Verification items for the finished model (mm, model axes). A direction names the side the tool comes from. Coordinates: 2 decimals unless noted, no trailing zeros. Loops run counter-clockwise (first coordinate to the right, second up) from the corner with the lowest first, then second, coordinate; pieces in that order, holes last. Notation, with made-up numbers: (-10, 80.25) - (4, 80.25) arc R37 cw to (4, 116.25) - close; hole circle Ø8 at (-24, -6). An arc over 180 degrees is marked (long way). One line per item, written item: value. Start each with the question number.
(1) Section check B-B (z = 5.5). Record the boundary of the cut face in (x, y), plus the area to 3 significant figures.
(2) Section check D-D (z = 1). Record the boundary of the cut face in (x, y).
(3) Gauge pin test, flat ends, axial feed: P1, Ø10, axis at x = 10.5, z = -14, coming from the +Y side; P2, Ø3, axis at x = -11.5, y = 1, coming from the -Z side; P3, Ø1.2, axis at y = 0, z = 12, coming from the -X side; P4, Ø1.5, axis at x = -20.06, y = 6.5, coming from the +Z side (3 decimals). Record the tip position at first contact, or that the pin passes through.
(4) Section check A-A (y = 6.5). Record the boundary of the cut face in (x, z), plus the area to 3 significant figures.
(5) Thickness scan on probe 1 along Z at (x, y) = (-10, 7); probe 2 along Y at (x, z) = (-4.5, -14.5); probe 3 along Y at (x, z) = (-20.06, 16.75). Record the ranges inside material, lowest first. Write a range as [from, to].
(6) Section check C-C (x = -6.8). Record the boundary of the cut face in (y, z), plus the area to 3 significant figures.
(7) Draft check along Z on faces 1 (the face through (-11, 0, -2.9)), 2 (the face through (-6.8, 9, -16.4)), 3 (the face through (-11, 0, 9.1)). Enter one of: +Z half, -Z half, draft (parallel to the pull), parting line (faces both ways), or undercut.
(8) Set-up check for faces 4 (the face through (-11, 0, 2.9)), 5 (the face through (-9, 4.7, -1)), 6 (the face through (-4, 7.9, 16)), 7 (the face through (-13, 7.9, 16)): record each of +Z, -Z, +X, -X, +Y, -Y from which the full face is reachable in a straight line by a thin tool's end or side.
```python
from build123d import *
from build123d.topology import SkipClean

# Parameters (mm, degrees)
EXTRUDE_1_DEPTH     = 18.5
SKETCH_2_W          = 6
SKETCH_2_H          = 5.8
SKETCH_2_H_2        = 9.4
SKETCH_2_W_2        = 12
SKETCH_2_H_3        = 20.2
CUT_EXTRUDE_1_DEPTH = 25.150569351
EXTRUDE_2_REACH     = 41.975
SKETCH_4_R          = 0.85
SKETCH_5_W          = 27.2
SKETCH_5_H          = 4.3
CUT_EXTRUDE_2_DEPTH = 43.825268242
SKETCH_6_W          = 27.2
SKETCH_6_H          = 0.5
CUT_EXTRUDE_3_DEPTH = 2


with BuildPart() as part:
    # 草图1 → 凸台-拉伸1 (new, symmetric)
    with BuildSketch(Plane.XY):
        with BuildLine():
            ThreePointArc((-11, 0), (-11.585786438, 1.414213562), (-13, 2))
            Line((-13, 2), (-13, 1.15))
            ThreePointArc((-13, 1.15), (-12.186827202, 0.813172798), (-11.85, 0))
            ThreePointArc((-11.85, 0), (-12.186827202, -0.813172798), (-13, -1.15))
            Line((-13, -1.15), (-13, -2))
            ThreePointArc((-13, -2), (-11.585786438, -1.414213562), (-11, 0))
        make_face()
        with BuildLine():
            Line((-13, 1.15), (-13, 2))
            ThreePointArc((-13, 2), (-15, 0), (-13, -2))
            Line((-13, -2), (-13, -1.15))
            ThreePointArc((-13, -1.15), (-14.15, 0), (-13, 1.15))
        make_face()
        with BuildLine():
            ThreePointArc((-11, 0), (-11.585786438, 1.414213562), (-13, 2))
            Line((-13, 2), (-13, 1.15))
            ThreePointArc((-13, 1.15), (-12.186827202, 0.813172798), (-11.85, 0))
            ThreePointArc((-11.85, 0), (-12.186827202, -0.813172798), (-13, -1.15))
            Line((-13, -1.15), (-13, -2))
            ThreePointArc((-13, -2), (-11.585786438, -1.414213562), (-11, 0))
        make_face()
        with BuildLine():
            Line((-13, 1.15), (-13, 2))
            ThreePointArc((-13, 2), (-15, 0), (-13, -2))
            Line((-13, -2), (-13, -1.15))
            ThreePointArc((-13, -1.15), (-14.15, 0), (-13, 1.15))
        make_face()
        with BuildLine():
            Line((13, 2), (-13, 2))
            ThreePointArc((-13, 2), (-11.585786438, 1.414213562), (-11, 0))
            ThreePointArc((-11, 0), (-11.585786438, -1.414213562), (-13, -2))
            Line((-13, -2), (13, -2))
            ThreePointArc((13, -2), (11, 0), (13, 2))
        make_face()
        with BuildLine():
            ThreePointArc((15, 0), (14.414213562, 1.414213562), (13, 2))
            Line((13, 2), (13, 1.15))
            ThreePointArc((13, 1.15), (13.813172798, 0.813172798), (14.15, 0))
            ThreePointArc((14.15, 0), (13.813172798, -0.813172798), (13, -1.15))
            Line((13, -1.15), (13, -2))
            ThreePointArc((13, -2), (14.414213562, -1.414213562), (15, 0))
        make_face()
        with BuildLine():
            Line((13, 1.15), (13, 2))
            ThreePointArc((13, 2), (11, 0), (13, -2))
            Line((13, -2), (13, -1.15))
            ThreePointArc((13, -1.15), (11.85, 0), (13, 1.15))
        make_face()
        with BuildLine():
            ThreePointArc((15, 0), (14.414213562, 1.414213562), (13, 2))
            Line((13, 2), (13, 1.15))
            ThreePointArc((13, 1.15), (13.813172798, 0.813172798), (14.15, 0))
            ThreePointArc((14.15, 0), (13.813172798, -0.813172798), (13, -1.15))
            Line((13, -1.15), (13, -2))
            ThreePointArc((13, -2), (14.414213562, -1.414213562), (15, 0))
        make_face()
        with BuildLine():
            Line((13, 1.15), (13, 2))
            ThreePointArc((13, 2), (11, 0), (13, -2))
            Line((13, -2), (13, -1.15))
            ThreePointArc((13, -1.15), (11.85, 0), (13, 1.15))
        make_face()
    extrude(amount=EXTRUDE_1_DEPTH, both=True)

    # 草图2 → 切除-拉伸1 (cut, through all)
    with SkipClean():  # the faces are left unmerged after this step: merging them gives an invalid solid
        with BuildSketch(Plane(origin=(0, 2, 0), x_dir=(1, 0, 0), z_dir=(0, 1, 0))):
            with Locations((-12, 0)):
                Rectangle(SKETCH_2_W, SKETCH_2_H)
            with Locations((-12, -13.8)):
                Rectangle(SKETCH_2_W, SKETCH_2_H_2)
            with Locations((-12, 13.8)):
                Rectangle(SKETCH_2_W, SKETCH_2_H_2)
            with Locations((9, 0)):
                Rectangle(SKETCH_2_W_2, SKETCH_2_H_3)
        extrude(amount=-CUT_EXTRUDE_1_DEPTH, mode=Mode.SUBTRACT)

    # 凸台-拉伸2: up to this face of the body (flat: up to its plane)
    extrude_2_end = Plane(part.part.faces().sort_by_distance((2.318945453, 0, -18.5))[0])
    # 草图4 → 凸台-拉伸2 (add, up to the picked face)
    with BuildSketch(Plane.XY.offset(18.5), mode=Mode.PRIVATE) as extrude_2_sk1:
        with BuildLine():
            Line((-10.789828689, 2.382780472), (-9, 2))
            Line((-9, 2), (8, 2))
            Line((8, 2), (-3.8, 7.9))
            Line((-3.8, 7.9), (-4.728768482, 7.9))
            ThreePointArc((-4.728768482, 7.9), (-6.8, 9), (-8.871231518, 7.9))
            Line((-8.871231518, 7.9), (-17.988768482, 7.9))
            ThreePointArc((-17.988768482, 7.9), (-20.06, 9), (-22.131231518, 7.9))
            Line((-22.131231518, 7.9), (-22.56, 7.9))
            Line((-22.56, 7.9), (-22.56, 4.9))
            Line((-22.56, 4.9), (-14.042229791, 3.078352979))
            ThreePointArc((-14.042229791, 3.078352979), (-12.320311008, 3.178131979), (-10.789828689, 2.382780472))
        make_face()
        with Locations((-20.06, 6.5)):
            Circle(SKETCH_4_R, mode=Mode.SUBTRACT)
        with Locations((-6.8, 6.5)):
            Circle(SKETCH_4_R, mode=Mode.SUBTRACT)
    extrude_2_tool1 = split(extrude(extrude_2_sk1.sketch, amount=-EXTRUDE_2_REACH, mode=Mode.PRIVATE), bisect_by=extrude_2_end, keep=Keep.BOTH, mode=Mode.PRIVATE)
    add(extrude_2_tool1.solids().sort_by(Axis((-8.777143, 5.120579, 18.5), (0, 0, -1)))[0])

    # 草图5 → 切除-拉伸2 (cut, through all)
    with SkipClean():  # the faces are left unmerged after this step: merging them gives an invalid solid
        with BuildSketch(Plane.ZY.offset(22.56)):
            with Locations((-0.7, 6.85)):
                Rectangle(SKETCH_5_W, SKETCH_5_H)
        extrude(amount=-CUT_EXTRUDE_2_DEPTH, mode=Mode.SUBTRACT)

    # 草图6 → 切除-拉伸3 (cut)
    with SkipClean():  # the faces are left unmerged after this step: merging them gives an invalid solid
        with BuildSketch(Plane.ZY.offset(22.56)):
            with Locations((-0.7, 4.7)):
                Rectangle(SKETCH_6_W, SKETCH_6_H)
        extrude(amount=-CUT_EXTRUDE_3_DEPTH, mode=Mode.SUBTRACT)


solid = part.part
```
Responses:
1. outline: (-20.56, 4.47) - (-14.04, 3.08) arc R3.25 cw to (-10.79, 2.38) - (-9, 2) - (-13, 2) arc R2 ccw to (-13, -2) - (3, -2) - (3, 2) - (8, 2) - (2.6, 4.7) - (-20.56, 4.7) - close; hole circle Ø2.3 at (-13, 0)
1. area: 121 mm²
2. outline: (-20.56, 4.47) - (-14.04, 3.08) arc R3.25 cw to (-10.79, 2.38) - (-9, 2) - (-9, -2) - (3, -2) - (3, 2) - (8, 2) - (2.6, 4.7) - (-20.56, 4.7) - close
3. P1: stops at y = 3.25
3. P2: stops at z = -9.1
3. P3: stops at x = -9
3. P4: passes through
4. outline: (-22.56, -18.5) - (-20.91, -18.5) - (-20.91, -14.3) - (-22.56, -14.3) - close; (-22.56, 12.9) - (-20.91, 12.9) - (-20.91, 18.5) - (-22.56, 18.5) - close; (-19.21, -18.5) - (-7.65, -18.5) - (-7.65, -14.3) - (-19.21, -14.3) - close; (-19.21, 12.9) - (-7.65, 12.9) - (-7.65, 18.5) - (-19.21, 18.5) - close; (-5.95, -18.5) - (-1, -18.5) - (-1, -14.3) - (-5.95, -14.3) - close; (-5.95, 12.9) - (-1, 12.9) - (-1, 18.5) - (-5.95, 18.5) - close
4. area: 178 mm²
5. probe 1: z = [-18.5, -14.3], [12.9, 18.5]
5. probe 2: y = [-2, 7.9]
5. probe 3: y = [4.37, 5.65], [7.35, 9]
6. outline: (-2, -18.5) - (5.65, -18.5) - (5.65, -14.3) - (4.7, -14.3) - (4.7, 12.9) - (5.65, 12.9) - (5.65, 18.5) - (-2, 18.5) - close; (7.35, -18.5) - (9, -18.5) - (9, -14.3) - (7.35, -14.3) - close; (7.35, 12.9) - (9, 12.9) - (9, 18.5) - (7.35, 18.5) - close
6. area: 273 mm²
7. face 1: undercut
7. face 2: draft
7. face 3: +Z half
8. face 4: -X, -Y
8. face 5: +X, -X, +Y
8. face 6: +Z, -Z, +X, +Y
8. face 7: +Z, -Z, +Y
